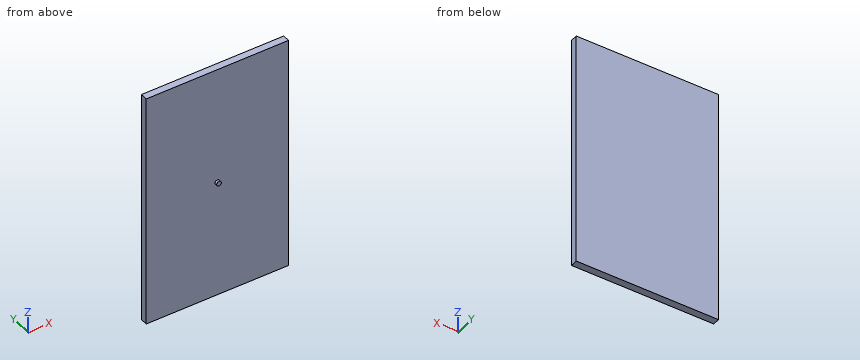
```python
from build123d import *

# Parameters (mm, degrees)
SKETCH8_W            = 600
SKETCH8_H            = 1000
BOSS_EXTRUDE9_DEPTH  = 30
SKETCH11_R           = 10
SKETCH11_R_2         = 5
BOSS_EXTRUDE12_DEPTH = 10
SKETCH12_R           = 10
BOSS_EXTRUDE13_DEPTH = 10


with BuildPart() as part:
    # Sketch8 → Boss-Extrude9 (new body)
    with BuildSketch(Plane(origin=(0, 0, 0), x_dir=(1, 0, 0), z_dir=(0, 1, 0))):
        Rectangle(SKETCH8_W, SKETCH8_H)
    extrude(amount=BOSS_EXTRUDE9_DEPTH)

    # Sketch11 → Boss-Extrude12 (add)
    with BuildSketch(Plane(origin=(0, 0, 0), x_dir=(1, 0, 0), z_dir=(0, 1, 0))):
        Circle(SKETCH11_R)
        Circle(SKETCH11_R_2, mode=Mode.SUBTRACT)
    extrude(amount=BOSS_EXTRUDE12_DEPTH)

    # Sketch12 → Boss-Extrude13 (add)
    with BuildSketch(Plane(origin=(0, 0, 0), x_dir=(-1, 0, 0), z_dir=(0, -1, 0))):
        with Locations(Location((0, 0, 0), (0, 0, 270))):
            Circle(SKETCH12_R)
    extrude(amount=BOSS_EXTRUDE13_DEPTH)


solid = part.part
```
The model under review builds one solid part; all positions refer to its coordinate system, in mm. Coordinates: 2 decimals unless noted, no trailing zeros. Write each loop counter-clockwise with the first axis right and the second up, starting at its lowest first coordinate (ties: lowest second). Pieces come first, ordered by that corner, then holes. Notation, with made-up numbers: (38, 72.5) -> (76, 72.5) arc R12 ccw to (76, 88.5) -> close; hole circle Ø9 at (35.25, -6). An arc over 180 degrees is marked (long way). One line per item, written item: value. Start each with the question number.
Q1. Add section B-B, the plane x = 0. Give the boundary of the cut face in (y, z), then the cut area to 3 significant figures.
Q2. Add section A-A, the plane z = 0. Give the boundary of the cut face in (x, y), then the cut area to 3 significant figures.
Q3. To check wall thickness, follow probe 1 along Y at (x, z) = (218.5, -226.5). State the ranges of the line that lie inside material, in increasing order.
Q4. Clearance check with a flat-ended pin moving along its axis: P1, Ø6, axis at x = 195.5, z = -72.5, coming from the -Y side. State where the tip first meets the part, or that it passes through.
Response:
1. outline: (-10, -10) -> (0, -10) -> (0, -500) -> (30, -500) -> (30, 500) -> (0, 500) -> (0, 10) -> (-10, 10) -> close
1. area: 30,200 mm²
2. outline: (-300, 0) -> (-10, 0) -> (-10, -10) -> (10, -10) -> (10, 0) -> (300, 0) -> (300, 30) -> (-300, 30) -> close
2. area: 18,200 mm²
3. probe 1: 0 to 30
4. P1: y = 0
